Can you work these out from the drawing? Everything is in mm from the part's minimum corner. A direction names the side the tool comes from. Give positions to 0.01 mm unless a question says otherwise; leave off trailing zeros. Write each loop counter-clockwise with the first axis right and the second up, starting at its lowest first coordinate (ties: lowest second). Pieces come first, ordered by that corner, then holes. Notation, with made-up numbers: (18, 10.25) - (40, 10.25) arc R21 ccw to (40, 28.25) - close; hole circle Ø8 at (18, -5). An arc over 180 degrees is marked (long way). Answer in a Markdown table with one row per item.
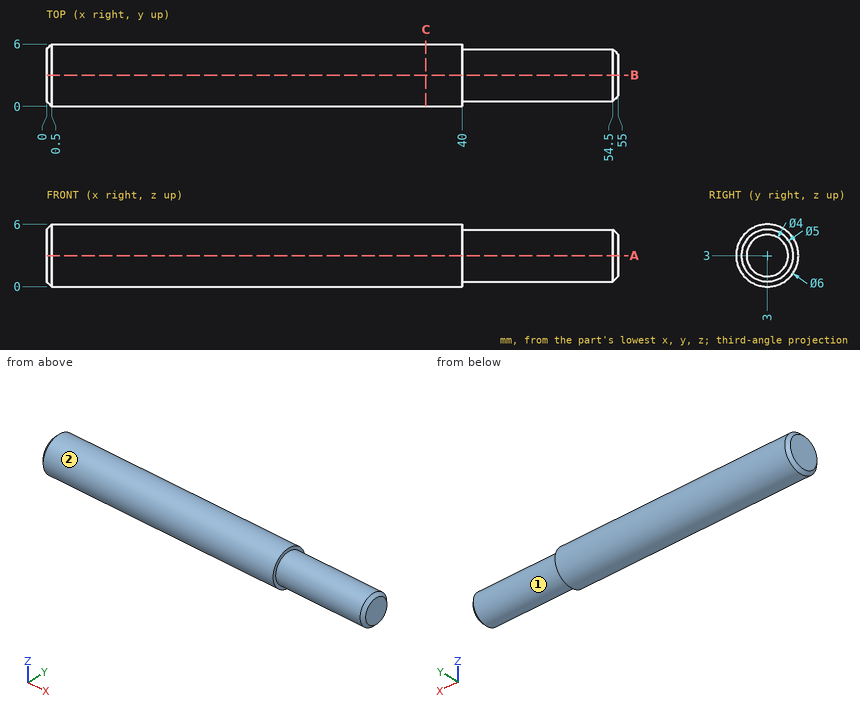
1) If I drill on line 1 (Z direction, x = 18.5, y = 2.85); line 2 (Z direction, x = 19, y = 0.3); line 3 (Y direction, x = 34.5, z = 4), over which ranges is the centre line in solid material (lowest first)?
Check values:
| item | result |
|---|---|
| line 1 | z = 0 to 6 |
| line 2 | z = 1.69 to 4.31 |
| line 3 | y = 0.17 to 5.83 |
2) Imagine slicing it at A-A (z = 3). List the corners of the cut face in (x, y) for me, then the cut area to 4 significant figures.
Check values:
| item | result |
|---|---|
| outline | (0, 0.5) - (0.5, 0) - (40, 0) - (40, 0.5) - (54.5, 0.5) - (55, 1) - (55, 5) - (54.5, 5.5) - (40, 5.5) - (40, 6) - (0.5, 6) - (0, 5.5) - close |
| area | 314.5 mm2 |
3) On a 3-axis mill with a long thin cutter (end or side, diameter ignored), from which of +Z, -Z, +X, -X, +Y, -Y can I reach the whole of each face in a straight line? I mean the marked faces 1 and 2. Say none if no direction works.
Check values:
| item | result |
|---|---|
| face 1 | +X |
| face 2 | +X, -X |
4) Imagine slicing it at C-C (x = 36.5). List the corners of the cut face in (y, z) for me.
Check values:
| item | result |
|---|---|
| outline | circle Ø6 at (3, 3) |
5) Will these pins go through, and if not, where does the flat tip stop? P1, Ø1, axis at y = 5, z = 5, coming from the +X side; P2, Ø3, axis at y = 5, z = 3.5, coming from the +X side.
Check values:
| item | result |
|---|---|
| P1 | stops at x = 54.67 |
| P2 | stops at x = 55 |
